from build123d import *

# Parameters (mm, degrees)
SKETCH_1_W               = 27
SKETCH_1_H               = 17
EXTRUDE_1_DEPTH          = 1
SKETCH_2_R               = 2.55
CUT_EXTRUDE_1_DEPTH      = 16.984367363
EXTRUDE_2_DEPTH          = 17
SKETCH_6_W               = 1.5
SKETCH_6_H               = 2
EXTRUDE_3_DEPTH          = 2
CHAMFER_1_SIZE           = 1
CUT_EXTRUDE_4_REACH      = 39.316
SKETCH_8_R               = 2
FILLET_1_R               = 3
SKETCH_9_W               = 7
SKETCH_9_H               = 13
EXTRUDE_4_DEPTH          = 1.5
SKETCH_7_R               = 1.35
CUT_EXTRUDE_5_DEPTH      = 10
CUT_EXTRUDE_6_REACH      = 41.373
FILLET_2_R               = 2.2
SKETCH_13_W              = 11.6
SKETCH_13_H              = 5.4
EXTRUDE_6_DEPTH          = 4
CUT_EXTRUDE_7_DEPTH      = 44.188540186
CUT_EXTRUDE_7_DEPTH_BACK = 44.188540186
SKETCH_14_OUTSIDE_W      = 46.664
SKETCH_14_OUTSIDE_H      = 47.664
SKETCH_14_OUTSIDE_W_2    = 27
SKETCH_14_OUTSIDE_H_2    = 5.5
EXTRUDE_7_DEPTH          = 3.5
EXTRUDE_7_DEPTH_BACK     = 10.5
SKETCH_16_W              = 5.6
SKETCH_16_H              = 1.5
SKETCH_16_W_2            = 4.4
SKETCH_16_W_3            = 12.2
EXTRUDE_8_DEPTH          = 2
EXTRUDE_9_DEPTH          = 2.5
CUT_EXTRUDE_8_REACH      = 54.983
SKETCH_18_W              = 5
SKETCH_18_H              = 9
EXTRUDE_START            = -1.5
SKETCH_19_R              = 3.726433752
SKETCH_19_R_2            = 1.35
SKETCH_19_W              = 24.8
SKETCH_19_H              = 1.288897449
EXTRUDE_10_DEPTH         = 1.5
FILLET_4_R               = 2


# Some blends are built 0.0001 mm under size
with BuildPart() as part:
    # 草图1 → 凸台-拉伸1 (new body)
    with BuildSketch(Plane.XY):
        Rectangle(SKETCH_1_W, SKETCH_1_H)
    extrude(amount=EXTRUDE_1_DEPTH)

    # 草图2 → 切除-拉伸1 (cut, through all)
    with BuildSketch(Plane.XY.offset(1)):
        with Locations((0, 4.125)):
            Circle(SKETCH_2_R)
        with Locations((0, -4.125)):
            Circle(SKETCH_2_R)
        with Locations((8.27, 4.125)):
            Circle(SKETCH_2_R)
        with Locations((8.27, -4.125)):
            Circle(SKETCH_2_R)
        with Locations((-8.27, 4.125)):
            Circle(SKETCH_2_R)
        with Locations((-8.27, -4.125)):
            Circle(SKETCH_2_R)
    extrude(amount=-CUT_EXTRUDE_1_DEPTH, mode=Mode.SUBTRACT)

    # 草图3 → 凸台-拉伸2 (add)
    with BuildSketch(Plane.XZ.offset(8.5)):
        Polygon((13.5, 0), (19, 0), (19, -28.5), (-13.5, -28.5), (-13.5, -30), (20.5, -30), (20.5, 1), (13.5, 1), align=None)
    extrude(amount=-EXTRUDE_2_DEPTH)

    # 草图6 → 凸台-拉伸3 (add, symmetric)
    with BuildSketch(Plane(origin=(0, 0, 0), x_dir=(1, 0, 0), z_dir=(0, 1, 0))):
        Polygon((19, 0), (19, 5), (14, 0), align=None)
        Polygon((19, 28.5), (14, 28.5), (19, 23.5), align=None)
        with Locations((18.25, 20)):
            Rectangle(SKETCH_6_W, SKETCH_6_H)
    extrude(amount=EXTRUDE_3_DEPTH, both=True)

    # 倒角1
    chamfer_1_edges = [part.edges().sort_by_distance(p)[0] for p in [
        (-13.5, 0, 0),
    ]]
    chamfer(chamfer_1_edges, length=CHAMFER_1_SIZE - 0.0001)  # a hair under: the kernel refuses the full size

    # 草图8 → 切除-拉伸4 (cut, up to next)
    with BuildSketch(Plane(origin=(0, 0, 0), x_dir=(-1, 0, 0), z_dir=(0, 0, -1)), mode=Mode.PRIVATE) as cut_extrude_4_sk1:
        Circle(SKETCH_8_R)
    cut_extrude_4_tool1 = extrude(cut_extrude_4_sk1.sketch, amount=-CUT_EXTRUDE_4_REACH, mode=Mode.PRIVATE) & part.part
    add(cut_extrude_4_tool1.solids().sort_by_distance((0, 0, 0))[0], mode=Mode.SUBTRACT)

    # 圆角1
    fillet_1_edges = [part.edges().sort_by_distance(p)[0] for p in [
        (20.5, 0, 1),
        (20.5, 0, -30),
        (19, 5.25, -28.5),
        (19, 5.25, 0),
        (19, -5.25, 0),
        (19, -5.25, -28.5),
    ]]
    fillet(fillet_1_edges, radius=FILLET_1_R)

    # 草图9 → 凸台-拉伸4 (add)
    with BuildSketch(Plane(origin=(0, 0, -30), x_dir=(-1, 0, 0), z_dir=(0, 0, -1))):
        with Locations((0, 6.5)):
            Rectangle(SKETCH_9_W, SKETCH_9_H)
    extrude(amount=-EXTRUDE_4_DEPTH)

    # 草图7 → 切除-拉伸5 (cut)
    with BuildSketch(Plane(origin=(0, 0, -30), x_dir=(-1, 0, 0), z_dir=(0, 0, -1))):
        with Locations((0, 10)):
            Circle(SKETCH_7_R)
        with Locations((-8.5, 2.7)):
            Circle(SKETCH_7_R)
        with Locations((8.5, 2.7)):
            Circle(SKETCH_7_R)
    extrude(amount=-CUT_EXTRUDE_5_DEPTH, mode=Mode.SUBTRACT)

    # 草图11 → 切除-拉伸6 (cut, up to next)
    with BuildSketch(Plane(origin=(0, 0, -30), x_dir=(-1, 0, 0), z_dir=(0, 0, -1)), mode=Mode.PRIVATE) as cut_extrude_6_sk1:
        with BuildLine():
            Line((13.5, -8.5), (13.5, 0))
            Line((13.5, 0), (-9, 0))
            ThreePointArc((-9, 0), (-15.01040764, -2.48959236), (-17.5, -8.5))
            Line((-17.5, -8.5), (13.5, -8.5))
        make_face()
    cut_extrude_6_tool1 = extrude(cut_extrude_6_sk1.sketch, amount=-CUT_EXTRUDE_6_REACH, mode=Mode.PRIVATE) & part.part
    add(cut_extrude_6_tool1.solids().sort_by_distance((1.149624, -4.397011, -30))[0], mode=Mode.SUBTRACT)

    # 圆角2
    fillet_2_edges = [part.edges().sort_by_distance(p)[0] for p in [
        (-3.5, 13, -29.25),
        (-3.5, 8.5, -29.25),
        (3.5, 13, -29.25),
        (3.5, 8.5, -29.25),
        (-13.5, 0, -29.25),
        (-13.5, 8.5, -29.25),
    ]]
    fillet(fillet_2_edges, radius=FILLET_2_R)

    # 草图13 → 凸台-拉伸6 (add)
    with BuildSketch(Plane(origin=(0, 0, -30), x_dir=(-1, 0, 0), z_dir=(0, 0, -1))):
        with Locations((0, 2.7)):
            Rectangle(SKETCH_13_W, SKETCH_13_H)
    extrude(amount=EXTRUDE_6_DEPTH)

    # 草图14 outside → 切除-拉伸7 (cut, two sides: drawn at the far end of the back side and taken through both)
    with BuildSketch(Plane(origin=(0, 8.5, 0), x_dir=(1, 0, 0), z_dir=(0, 1, 0)).offset(-CUT_EXTRUDE_7_DEPTH_BACK)):
        with Locations((3.5, 16.5)):
            Rectangle(SKETCH_14_OUTSIDE_W, SKETCH_14_OUTSIDE_H)
        with Locations((0, 31.25)):
            Rectangle(SKETCH_14_OUTSIDE_W_2, SKETCH_14_OUTSIDE_H_2, mode=Mode.SUBTRACT)
    extrude(amount=CUT_EXTRUDE_7_DEPTH + CUT_EXTRUDE_7_DEPTH_BACK, mode=Mode.SUBTRACT)

    # 草图15 → 凸台-拉伸7 (add, two sides: drawn at the far end of the back side and taken through both)
    with BuildSketch(Plane.XZ.offset(-EXTRUDE_7_DEPTH_BACK)):
        Polygon((-19.25, -14.25), (-19.25, -30), (-11.3, -30), (-11.3, -28.5), (-17.75, -28.5), (-17.75, -19.35), (-16.15, -19.35), (-16.15, -17.35), (-17.75, -17.35), (-17.75, -16.25), (-15.25, -16.25), (-15.25, -14.25), align=None)
        Polygon((17.75, -28.5), (13.5, -28.5), (13.5, -30), (19.25, -30), (19.25, -14.25), (15.25, -14.25), (15.25, -16.25), (17.75, -16.25), (17.75, -17.35), (16.15, -17.35), (16.15, -19.35), (17.75, -19.35), align=None)
    extrude(amount=EXTRUDE_7_DEPTH + EXTRUDE_7_DEPTH_BACK)

    # 草图16 → 凸台-拉伸8 (add)
    with BuildSketch(Plane(origin=(0, 8.5, 0), x_dir=(1, 0, 0), z_dir=(0, 1, 0))):
        with Locations((-8.5, 29.25)):
            Rectangle(SKETCH_16_W, SKETCH_16_H)
        with Locations((-3.5, 29.25)):
            Rectangle(SKETCH_16_W_2, SKETCH_16_H)
        with Locations((7.4, 29.25)):
            Rectangle(SKETCH_16_W_3, SKETCH_16_H)
    extrude(amount=EXTRUDE_8_DEPTH)

    # 草图17 → 凸台-拉伸9 (add, symmetric)
    with BuildSketch(Plane(origin=(0, 3.5, 0), x_dir=(-1, 0, 0), z_dir=(0, -1, 0))):
        Polygon((17.75, 25.275), (14.525, 28.5), (17.75, 28.5), align=None)
        Polygon((-17.75, 25.275), (-17.75, 28.5), (-14.525, 28.5), align=None)
    extrude(amount=EXTRUDE_9_DEPTH, both=True)

    # 切除-拉伸8: up to this face of the body (flat: up to its plane)
    cut_extrude_8_end = Plane(part.part.faces().sort_by_distance((17.75, 3.5, -16.8))[0])
    # 草图18 → 切除-拉伸8 (cut, up to the picked face)
    with BuildSketch(Plane.ZY.offset(19.25), mode=Mode.PRIVATE) as cut_extrude_8_sk1:
        with Locations((-19.85, 3.5)):
            Rectangle(SKETCH_18_W, SKETCH_18_H)
    cut_extrude_8_tool1 = split(extrude(cut_extrude_8_sk1.sketch, amount=-CUT_EXTRUDE_8_REACH, mode=Mode.PRIVATE), bisect_by=cut_extrude_8_end, keep=Keep.BOTH, mode=Mode.PRIVATE)
    add(cut_extrude_8_tool1.solids().sort_by(Axis((-19.25, 3.5, -19.85), (1, 0, 0)))[0], mode=Mode.SUBTRACT)

    # 草图19 → 凸台-拉伸10 (add)
    # profile 1 of 2: a face of its own
    with BuildSketch(Plane.XY.offset(-28.5).offset(EXTRUDE_START)):
        with Locations((0, 10)):
            Circle(SKETCH_19_R)
        with Locations((0, 10)):
            Circle(SKETCH_19_R_2, mode=Mode.SUBTRACT)
    # profile 2 of 2: a face of its own
    with BuildSketch(Plane.XY.offset(-28.5).offset(EXTRUDE_START)):
        with Locations((1.1, -0.644448725)):
            Rectangle(SKETCH_19_W, SKETCH_19_H)
    extrude(amount=EXTRUDE_10_DEPTH)

    # 圆角4
    # the kernel refuses this fillet: 2 mm, written as the material it adds along each edge
    with BuildSketch(Plane(origin=(13.5, -1.288897449, -28.5), x_dir=(0, -1, 0), z_dir=(0, 0, -1))) as fillet_4_piece_1:
        with BuildLine():
            CenterArc((FILLET_4_R, FILLET_4_R), FILLET_4_R, 180, 90)
            Line((0, FILLET_4_R), (0, 0))
            Line((0, 0), (FILLET_4_R, 0))
        make_face()
    extrude(amount=1.5)
    with BuildSketch(Plane(origin=(17.75, 1, -28.5), x_dir=(-1, 0, 0), z_dir=(0, 1, 0)), Plane(origin=(-17.75, 6, -28.5), x_dir=(1, 0, 0), z_dir=(0, -1, 0)), Plane(origin=(-17.75, 10.5, -28.5), x_dir=(1, 0, 0), z_dir=(0, -1, 0)), Plane(origin=(17.75, -3.5, -28.5), x_dir=(-1, 0, 0), z_dir=(0, 1, 0))) as fillet_4_piece_2:
        with BuildLine():
            CenterArc((FILLET_4_R, FILLET_4_R), FILLET_4_R, 180, 90)
            Line((0, FILLET_4_R), (0, 0))
            Line((0, 0), (FILLET_4_R, 0))
        make_face()
    extrude(amount=9.5)
    with BuildSketch(Plane(origin=(-3.692737265, 10.5, -28.5), x_dir=(-1, 0, 0), z_dir=(0, 0, -1))) as fillet_4_piece_3:
        with BuildLine():
            CenterArc((1.459159814, 2), FILLET_4_R, 205.88535786, 64.11464214)
            ThreePointArc((-0.340178937, 1.126856222), (-0.125315404, 0.576944648), (0, 0))
            Line((0, 0), (1.459159814, 0))
        make_face()
    extrude(amount=1.5)
    with BuildSketch(Plane(origin=(3.692737265, 10.5, -28.5), x_dir=(-0.28900142054358374, 0.9573286681823493, 0), z_dir=(0, 0, -1))) as fillet_4_piece_4:
        with BuildLine():
            CenterArc((1.492958077, 1.974898363), FILLET_4_R, 196.798181975, 64.11464214)
            Line((-0.421699259, 1.396895522), (0, 0))
            ThreePointArc((0, 0), (0.588541981, 0.046769794), (1.177083962, 0))
        make_face()
    extrude(amount=1.5)
    with BuildSketch(Plane(origin=(-5.8, 0, -30), x_dir=(0, -1, 0), z_dir=(1, 0, 0))) as fillet_4_piece_5:
        with BuildLine():
            CenterArc((2, 1.869313554), FILLET_4_R, 180, 69.172765444)
            Line((0, 1.869313554), (0, 0))
            Line((0, 0), (1.288897449, 0))
        make_face()
    extrude(amount=11.6)
    with BuildSketch(Plane(origin=(-11.3, -1.288897449, -30), x_dir=(1, 0, 0), z_dir=(0, 0, 1))) as fillet_4_piece_6:
        with BuildLine():
            CenterArc((FILLET_4_R, -FILLET_4_R), FILLET_4_R, 90, 90)
            Line((0, -FILLET_4_R), (0, 0))
            Line((0, 0), (FILLET_4_R, 0))
        make_face()
    extrude(amount=1.5)
    # the kernel refuses this fillet: 2 mm, written as the material it takes off along each edge
    with BuildSketch(Plane(origin=(19.25, 15.5, -30), x_dir=(-1, 0, 0), z_dir=(0, -1, 0))) as fillet_4_2_piece_1:
        with BuildLine():
            CenterArc((FILLET_4_R, -FILLET_4_R), FILLET_4_R, 90, 90)
            Line((0, -FILLET_4_R), (0, 0))
            Line((0, 0), (FILLET_4_R, 0))
        make_face()
    extrude(amount=24, mode=Mode.SUBTRACT)
    with BuildSketch(Plane(origin=(-19.25, 15.5, -30), x_dir=(1, 0, 0), z_dir=(0, -1, 0))) as fillet_4_2_piece_2:
        with BuildLine():
            CenterArc((FILLET_4_R, FILLET_4_R), FILLET_4_R, 180, 90)
            Line((0, FILLET_4_R), (0, 0))
            Line((0, 0), (FILLET_4_R, 0))
        make_face()
    extrude(amount=24, mode=Mode.SUBTRACT)


solid = part.part
Geometry: final body of the model. Coordinates: model frame, mm. A direction names the side the tool comes from. Give positions to 0.01 mm unless a question says otherwise; leave off trailing zeros. Loops run counter-clockwise (first coordinate to the right, second up) from the corner with the lowest first, then second, coordinate; pieces in that order, holes last. Notation, with made-up numbers: M 3,82.5 L 60,82.5 A26 cw 60,105.5 Z; hole C 13,43 d1. An arc over 180 degrees is marked long. Put each result on its own line as item: value. Start each with the question number.
1) Cut plane C-C (y = 2.7). Give the number of separate pieces and of enclosed holes in the cut face, then the cut area to 3 significant figures.
2) Ray query, line 1 along X through (y, z) = (0, -25); line 2 along Y through (x, z) = (8.5, -28.95); line 3 along Z through (x, y) = (-17, -1.75). Return the intervals inside material, ascending.
3) Contact query for flat-ended pins moving along their axis: pin 1 (4 mm diameter, centred on x = 8, z = -30.5, fed in from +Y); pin 2 (3.5 mm diameter, centred on x = -15.5, z = -26.5, fed in from +Y); pin 3 (0.8 mm diameter, centred on y = 10, z = -29.5, fed in from -X). Output: stop coordinate, or through.
4) Cut plane A-A (x = -8.5). Output: boundary loops of the cut face in (y, z).
5) Access query for faces 4 (the flat face through (-18, 8, -19)), 5 (the flat face through (16.5, 6, -27.3)), 6 (the cylindrical face through (-17.18, -1.22, -27.9)), 7 (the flat face through (-16.16, 3.535, -26.865)), 8 (the cylindrical face through (-0.02, 11.35, -29.26)). Directions: +Z, -Z, +X, -X, +Y, -Y. A direction counts if a zero-diameter tool reaches every point of the face in a straight line with its end or side. Return the directions, or none.
6) Pull-direction query (Z, two-part tool) for faces 1 (the flat face through (-15.25, 4, -15)), 2 (the cylindrical face through (-0.081, -0.344, -30.748)), 3 (the flat face through (16.115, 3.465, -26.91)); classes: pulls with the +Z half, pulls with the -Z half, needs draft (parallel to the pull), parting line crosses it, or undercut.
7) Cut plane D-D (y = -2). Output: boundary loops of the cut face in (x, z).
8) Cut plane B-B (y = 7). Output: boundary loops of the cut face in (x, z), then the cut area to 3 significant figures.
Verdict:
1. separate pieces: 4
1. enclosed holes: 0
1. area: 150 mm2
2. line 1: -19.25 to -17.75, 17.75 to 19.25
2. line 2: -1.29 to 1.35, 4.05 to 10.5
2. line 3: -30 to -28.06, -19.35 to -17.35, -16.25 to -14.25
3. pin 1: y = 10.5
3. pin 2: y = 6
3. pin 3: x = -18.92
4. outline: M -1.29,-30 L 1.35,-30 L 1.35,-28.5 L -1.29,-28.5 Z; M 4.05,-30 L 10.5,-30 L 10.5,-28.5 L 4.05,-28.5 Z
5. face 4: -X
5. face 5: +Y
5. face 6: -Y
5. face 7: +Y, -Y
5. face 8: +Z, -Z
6. face 1: needs draft
6. face 2: pulls with the -Z half
6. face 3: undercut
7. outline: M -19.25,-28 A2 ccw -17.25,-30 L -10.83,-30 L -10.83,-28.5 L -15.75,-28.5 A2 cw -17.75,-26.5 L -17.75,-19.35 L -16.15,-19.35 L -16.15,-17.35 L -17.75,-17.35 L -17.75,-16.25 L -15.25,-16.25 L -15.25,-14.25 L -19.25,-14.25 Z; M 13.03,-30 L 17.25,-30 A2 ccw 19.25,-28 L 19.25,-14.25 L 15.25,-14.25 L 15.25,-16.25 L 17.75,-16.25 L 17.75,-17.35 L 16.15,-17.35 L 16.15,-19.35 L 17.75,-19.35 L 17.75,-26.5 A2 cw 15.75,-28.5 L 13.03,-28.5 Z
8. outline: M -19.25,-28 A2 ccw -17.25,-30 L 17.25,-30 A2 ccw 19.25,-28 L 19.25,-14.25 L 15.25,-14.25 L 15.25,-16.25 L 17.75,-16.25 L 17.75,-26.5 A2 cw 15.75,-28.5 L -15.75,-28.5 A2 cw -17.75,-26.5 L -17.75,-22.35 L -19.25,-22.35 Z; M -19.25,-17.35 L -17.75,-17.35 L -17.75,-16.25 L -15.25,-16.25 L -15.25,-14.25 L -19.25,-14.25 Z
8. area: 103 mm2
